Read the model definition and answer for the solid it produces. Units are mm, in the model's axes. A direction names the side the tool comes from. Round coordinates to 2 decimals unless told otherwise and drop trailing zeros. Order: outer loops, then holes, each group sorted by start corner. A loop starts at its lowest first (then second) coordinate and runs counter-clockwise, first axis right, second up. Notation, with made-up numbers: M -4,39 L 39,39 A30 cw 39,77 Z; hole C 12.5,29.5 d7. An arc over 180 degrees is marked long. Answer as CSV lines item,"result".
```python
from build123d import *
from build123d.topology import SkipClean

# Parameters (mm, degrees)
SKETCH_1_R          = 3.333333333
SKETCH_1_R_2        = 5
EXTRUDE_1_DEPTH     = 5
EXTRUDE_START       = 6
SKETCH_6_R          = 5
EXTRUDE_5_DEPTH     = 6
EXTRUDE_START_2     = 2
SKETCH_7_R          = 2
EXTRUDE_6_DEPTH     = 2
SKETCH_9_R          = 2
CUT_EXTRUDE_3_DEPTH = 79.745912397
EXTRUDE_START_3     = -11
SKETCH_10_R         = 5
SKETCH_10_R_2       = 2
EXTRUDE_7_DEPTH     = 11
FILLET_2_R          = 10
SCALE_1_SCALE       = 1.5
SKETCH_11_R         = 3
CUT_EXTRUDE_4_DEPTH = 6
EXTRUDE_START_4     = -15
SKETCH_12_R         = 3
SKETCH_12_R_2       = 2.6
EXTRUDE_8_DEPTH     = 15
SKETCH_13_R         = 5
CUT_EXTRUDE_5_DEPTH = 5.6
EXTRUDE_START_5     = -4.4
SKETCH_15_R         = 5
SKETCH_15_R_2       = 3
EXTRUDE_9_DEPTH     = 3.1
SKETCH_16_R         = 6
CUT_EXTRUDE_6_DEPTH = 0.4


with BuildPart() as part:
    # 草图1 → 凸台-拉伸1 (new body)
    with BuildSketch(Plane.XY):
        with BuildLine():
            Line((14.059772875, 0), (63.798276921, 0))
            ThreePointArc((63.798276921, 0), (70.56109353, -5.193259423), (67.289321258, -13.067339568))
            Line((67.289321258, -13.067339568), (32.61880944, -33.016164352))
            ThreePointArc((32.61880944, -33.016164352), (27.731011729, -33.808057978), (23.542094163, -31.167862607))
            Line((23.542094163, -31.167862607), (8.474101936, -11.219037824))
            ThreePointArc((8.474101936, -11.219037824), (7.793463564, -3.88016545), (14.059772875, 0))
        make_face()
        with Locations((29.127765103, -24.948824784)):
            Circle(SKETCH_1_R, mode=Mode.SUBTRACT)
        with Locations((61.298276921, -7.5)):
            Circle(SKETCH_1_R_2, mode=Mode.SUBTRACT)
    extrude(amount=EXTRUDE_1_DEPTH)

    # 草图6 → 凸台-拉伸5 (add)
    with SkipClean():  # the faces are left unmerged after this step: merging them gives an invalid solid
        with BuildSketch(Plane(origin=(0, 0, 0), x_dir=(-1, 0, 0), z_dir=(0, 0, -1)).offset(EXTRUDE_START)):
            with BuildLine():
                Line((-67.289321258, -13.067339568), (-55.111154239, -20.074450433))
                Line((-55.111154239, -20.074450433), (-49.187018483, -12.783115053))
                Line((-49.187018483, -12.783115053), (-53.134085027, 0))
                Line((-53.134085027, 0), (-63.798276921, 0))
                ThreePointArc((-63.798276921, 0), (-70.56109353, -5.193259423), (-67.289321258, -13.067339568))
            make_face()
            with Locations((-61.298276921, -7.5)):
                Circle(SKETCH_6_R, mode=Mode.SUBTRACT)
        extrude(amount=-EXTRUDE_5_DEPTH)

    # 草图7 → 凸台-拉伸6 (add)
    with SkipClean():  # the faces are left unmerged after this step: merging them gives an invalid solid
        with BuildSketch(Plane(origin=(0, 0, 0), x_dir=(-1, 0, 0), z_dir=(0, 0, -1)).offset(EXTRUDE_START_2)):
            with BuildLine():
                Line((-14.059772875, 0), (-25.059772875, 0))
                Line((-25.059772875, 0), (-26.163863889, -10))
                Line((-26.163863889, -10), (-13.040056703, -17.263999238))
                Line((-13.040056703, -17.263999238), (-8.474101936, -11.219037824))
                ThreePointArc((-8.474101936, -11.219037824), (-7.793463564, -3.88016545), (-14.059772875, 0))
            make_face()
            with Locations((-16.298276921, -7.5)):
                Circle(SKETCH_7_R, mode=Mode.SUBTRACT)
        extrude(amount=-EXTRUDE_6_DEPTH)

    # 草图9 → 切除-拉伸3 (cut, through all)
    with SkipClean():  # the faces are left unmerged after this step: merging them gives an invalid solid
        with BuildSketch(Plane(origin=(0, 0, 0), x_dir=(-1, 0, 0), z_dir=(0, 0, -1))):
            with Locations((-16.298276921, -7.5)):
                Circle(SKETCH_9_R)
        extrude(amount=-CUT_EXTRUDE_3_DEPTH, mode=Mode.SUBTRACT)

    # 草图10 → 凸台-拉伸7 (add)
    with BuildSketch(Plane.XY.offset(5).offset(EXTRUDE_START_3)):
        with Locations((61.298276921, -7.5)):
            Circle(SKETCH_10_R)
        with Locations((61.298276921, -7.5)):
            Circle(SKETCH_10_R_2, mode=Mode.SUBTRACT)
    extrude(amount=EXTRUDE_7_DEPTH)

    # 圆角2
    fillet_2_edges = [part.edges().sort_by_distance(p)[0] for p in [
        (49.187018483, -12.783115053, -3),
        (26.163863889, -10, -1),
    ]]
    fillet(fillet_2_edges, radius=FILLET_2_R)


with BuildPart() as part_1:
    # 缩放比例1: scaled about (40.486651363, -11.642315259, 1.295457426)
    add(part.part.scale(SCALE_1_SCALE).moved(Location((-20.243325682, 5.82115763, -0.647728713))))

    # 草图11 → 切除-拉伸4 (cut)
    with BuildSketch(Plane(origin=(0, 0, -3.647728713), x_dir=(-1, 0, 0), z_dir=(0, 0, -1))):
        with BuildLine():
            Line((-17.346333632, 5.82115763), (-17.905962845, 0.752470301))
            ThreePointArc((-17.905962845, 0.752470301), (-15.308702596, -15.14882708), (-4.859629901, -27.41316151))
            Line((-4.859629901, -27.41316151), (7.532172777, -11.007399106))
            ThreePointArc((7.532172777, -11.007399106), (8.553130335, 0.000909454), (-0.846333632, 5.82115763))
            Line((-0.846333632, 5.82115763), (-17.346333632, 5.82115763))
        make_face()
        with Locations((-4.2040897, -5.42884237)):
            Circle(SKETCH_11_R, mode=Mode.SUBTRACT)
    extrude(amount=-CUT_EXTRUDE_4_DEPTH, mode=Mode.SUBTRACT)

    # 草图12 → 凸台-拉伸8 (add)
    with BuildSketch(Plane.XY.offset(6.852271287).offset(EXTRUDE_START_4)):
        with Locations((71.7040897, -5.42884237)):
            Circle(SKETCH_12_R)
        with Locations((71.7040897, -5.42884237)):
            Circle(SKETCH_12_R_2, mode=Mode.SUBTRACT)
    extrude(amount=EXTRUDE_8_DEPTH)

    # 草图13 → 切除-拉伸5 (cut)
    with BuildSketch(Plane.XY.offset(6.852271287)):
        with Locations((71.7040897, -5.42884237)):
            Circle(SKETCH_13_R)
    extrude(amount=-CUT_EXTRUDE_5_DEPTH, mode=Mode.SUBTRACT)

    # 草图15 → 凸台-拉伸9 (add)
    with BuildSketch(Plane(origin=(0, 0, -0.647728713), x_dir=(-1, 0, 0), z_dir=(0, 0, -1)).offset(EXTRUDE_START_5)):
        with Locations((-23.448321972, -31.602079546)):
            Circle(SKETCH_15_R)
        with Locations((-23.448321972, -31.602079546)):
            Circle(SKETCH_15_R_2, mode=Mode.SUBTRACT)
    extrude(amount=-EXTRUDE_9_DEPTH)

    # 草图16 → 切除-拉伸6 (cut)
    with BuildSketch(Plane(origin=(0, 0, -0.647728713), x_dir=(-1, 0, 0), z_dir=(0, 0, -1))):
        with Locations((-23.448321972, -31.602079546)):
            Circle(SKETCH_16_R)
    extrude(amount=-CUT_EXTRUDE_6_DEPTH, mode=Mode.SUBTRACT)


solid = part_1.part
```
Item 1: A cutting plane is placed at A-A, the plane y = -33. Determine the outline of the cut face in (x, z), and give its area (3 significant figures).
Ans:
outline,"M 9.08,-0.65 L 17.61,-0.65 L 17.61,-0.25 L 18.65,-0.25 L 18.65,3.75 L 20.79,3.75 L 20.79,6.85 L 9.08,6.85 Z; M 26.1,3.75 L 28.25,3.75 L 28.25,-0.25 L 29.28,-0.25 L 29.28,-0.65 L 47.29,-0.65 L 47.29,6.85 L 26.1,6.85 Z"
area,"227 mm2"
Item 2: A cutting plane is placed at D-D, the plane y = -23. Determine the outline of the cut face in (x, z).
Ans:
outline,"M 1.53,2.35 L 10.03,2.35 L 10.03,-0.65 L 61.37,-0.65 L 61.37,-9.65 L 64.67,-9.65 L 64.67,6.85 L 1.53,6.85 Z"
Item 3: A cutting plane is placed at B-B, the plane x = 72.5. Determine the outline of the cut face in (y, z).
Ans:
outline,"M -18.49,-9.65 L -8.32,-9.65 L -8.32,-8.15 L -7.9,-8.15 L -7.9,1.25 L -10.37,1.25 L -10.37,6.85 L -18.49,6.85 Z; M -2.95,-8.15 L -2.54,-8.15 L -2.54,-9.65 L 5.82,-9.65 L 5.82,6.85 L -0.49,6.85 L -0.49,1.25 L -2.95,1.25 Z"
Item 4: Determine the mould class of faces 4 (the face through (85.547, -1.783, -1.513)), 5 (the face through (60.54, -21.97, -5.21)), 6 (the face through (34, -19, -0.648)), 7 (the face through (74.566, -4.528, -8.908)) for opening direction X: +X half, -X half, draft (parallel to the pull), parting line (faces both ways), or undercut.
Ans:
face 4,"+X half"
face 5,"-X half"
face 6,"draft"
face 7,"undercut"
Item 5: Flat-ended cylindrical pins translate along their axes: pin 1 (8 mm diameter, centred on x = 71.7, y = -5.43, fed in from +Z); pin 2 (8 mm diameter, centred on x = 13, y = -30, fed in from -Z); pin 3 (8 mm diameter, centred on y = -19.5, z = -5.5, fed in from -X). Find the tip coordinate at first contact, or state that the pin passes through.
Ans:
pin 1,"z = 1.25"
pin 2,"z = -0.65"
pin 3,"x = 56.23"
Item 6: A tool of negligible diameter and unlimited length cuts with its end or side. For faces 1 (the face through (17.622, 3.322, 0.831)), 2 (the face through (74, -8, 1.252)), 3 (the face through (71.2, -2.7, -8.148)), from which of +Z, -Z, +X, -X, +Y, -Y can it reach the whole face along a straight path? Write none if from no direction.
Ans:
face 1,"-Z, -X"
face 2,"+Z"
face 3,"-Z"
Item 7: Find the intervals of material crossed by probe 1 along Y at (x, z) = (21, 1.25); probe 2 along Z at (x, y) = (13, -25.5); probe 3 along Z at (x, y) = (-2, -16.5), in increasing order. Write a range as [from, to].
Ans:
probe 1,"[-44.81, -35.96], [-27.24, 5.82]"
probe 2,"[-0.65, 6.85]"
probe 3,"[2.35, 6.85]"
Item 8: A cutting plane is placed at C-C, the plane z = 5. Determine the outline of the cut face in (x, y).
Ans:
outline,"M -7.53,-11.01 L 15.07,-40.93 A10.5 ccw 28.68,-43.7 L 80.69,-13.78 A10.5 ccw 75.45,5.82 L 0.85,5.82 A10.5 ccw Z; hole C 4.2,-5.43 d6; hole C 23.45,-31.6 d6; hole C 71.7,-5.43 d10"
